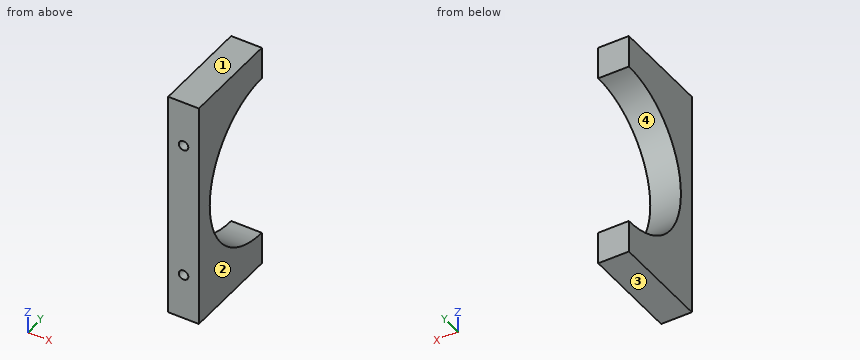
Autodesk Inventor part; units mm, degrees
ref_plane "YZ Plane" through (0, 0, 0) normal (1, 0, 0) x (0, 1, 0)
ref_plane "XZ Plane" through (0, 0, 0) normal (0, 1, 0) x (-1, 0, 0)
ref_plane "XY Plane" through (0, 0, 0) normal (0, 0, 1) x (1, 0, 0)
sketch "스케치1" plane through (0, 0, 0) normal (1, 0, 0) x (0, 1, 0)
  line L0 (0, 0) -> (27, 0)
  line L1 (27, -60) -> (0, -60)
  line L2 (0, -60) -> (0, 0)
  arc A0 (27, -8.5) -> (27, -51.5) centre (27, -30) ccw
  line L3 (27, 0) -> (27, -8.5)
  line L4 (27, -51.5) -> (27, -60)
  dimension "d0" = 27
  dimension "d3" = 60
  dimension "d4" = 27
  dimension "d5" = 21.5
  dimension "d6" = 27
  dimension "d7" = 30
extrude "돌출1" add sketch "스케치1" along normal blind 8
sketch "스케치2" plane through (0, 0, -60) normal (0, -1, 0) x (1, 0, 0)
  line L0 (0, 0) -> (0, 60)
  line L1 (0, 0) -> (8, 0)
  line L2 (8, 60) -> (8, 0)
  line L3 (0, 60) -> (8, 60)
  line L4 (0, 60) -> (0, 51.5)
  line L5 (0, 60) -> (8, 60)
  line L6 (8, 51.5) -> (8, 60)
  line L7 (0, 51.5) -> (8, 51.5)
  line L8 (0, 8.5) -> (0, 0)
  line L9 (0, 8.5) -> (8, 8.5)
  line L10 (8, 0) -> (8, 8.5)
  line L11 (0, 0) -> (8, 0)
  circle A0 centre (4, 48) radius 1.25
  circle A1 centre (4, 12) radius 1.25
  dimension "d10" = 2.5
  dimension "d11" = 2.5
  dimension "d12" = 4
  dimension "d13" = 4
  dimension "d14" = 12
  dimension "d15" = 12
extrude "돌출2" cut sketch "스케치2" against normal blind 9 contours A0 | A1
sketch "스케치3" plane through (0, 0, -60) normal (0, -1, 0) x (1, 0, 0)
  circle A0 centre (4, 48) radius 1.25
  circle A1 centre (4, 12) radius 1.25
  line L0 (0, 0) -> (0, 60)
  line L1 (0, 0) -> (8, 0)
  line L2 (8, 60) -> (8, 0)
  line L3 (0, 60) -> (8, 60)
extrude "돌출3" cut sketch "스케치3" against normal blind 1
properties part number "모터받침대" material "ABS 플라스틱"
CAD build for the part. Positions are in the model's coordinates, mm. Face numbers are marked on the shaded views. Coordinates: 2 decimals unless noted, no trailing zeros. Write each loop counter-clockwise with the first axis right and the second up, starting at its lowest first coordinate (ties: lowest second). Pieces come first, ordered by that corner, then holes. Notation, with made-up numbers: (68, 40.25) -> (87, 40.25) arc R23 ccw to (87, 65.25) -> close; hole circle Ø5 at (-27.75, 13.5). An arc over 180 degrees is marked (long way). Return JSON: item names as keys, results as strings. Group by question number.
Q1. Cut at C-C, the plane z = -12. Give the cut face in (x, y).
Q2. Flat gauge pins, fed straight in: pin 1 (2 mm diameter, centred on x = 2.5, y = 23, fed in from +Z); pin 2 (2 mm diameter, centred on x = 4, z = -48, fed in from +Y); pin 3 (0.8 mm diameter, centred on x = 4, z = -47.5, fed in from -Y). Where does each tip first touch, or does it go through?
Q3. Drill centre lines: line 1 (Z direction, x = 4, y = 3.25); line 2 (Z direction, x = 4, y = 7.25); line 3 (Z direction, x = 7.75, y = 24.5). Where is each one in solid material? Low to high.
Q4. Cut at B-B, the plane x = 1.25. Give the cut face in (y, z).
Q5. Cut at D-D, the plane y = 24.75. Give the cut face in (x, z), then the cut area to 3 significant figures.
Q6. Cut at A-A, the plane y = 20.5. Give the cut face in (x, z), then the cut area to 3 significant figures.
Q7. Pull direction Z, two halves, no side cores. Call the marked faces 1, 2, 3 and 4: released by +Z, released by -Z, zero draft, split by the parting line, or undercut.
Returned:
{
 "1": {"outline": "(0, 1) -> (2.75, 1) -> (2.75, 9) -> (5.25, 9) -> (5.25, 1) -> (8, 1) -> (8, 15.24) -> (0, 15.24) -> close"},
 "2": {"pin 1": "stops at z = 0", "pin 2": "stops at y = 16.94", "pin 3": "stops at y = 9"},
 "3": {"line 1": "z = -60 to -49.25, -46.75 to -13.25, -10.75 to 0", "line 2": "z = -60 to -49.25, -46.75 to -38.5, -21.5 to -13.25, -10.75 to 0", "line 3": "z = -60 to -51.35, -8.65 to 0"},
 "4": {"outline": "(1, -60) -> (27, -60) -> (27, -51.5) arc R21.5 cw to (27, -8.5) -> (27, 0) -> (1, 0) -> close"},
 "5": {"outline": "(0, -60) -> (8, -60) -> (8, -51.38) -> (0, -51.38) -> close; (0, -8.62) -> (8, -8.62) -> (8, 0) -> (0, 0) -> close", "area": "138 mm2"},
 "6": {"outline": "(0, -60) -> (8, -60) -> (8, -50.49) -> (0, -50.49) -> close; (0, -9.51) -> (8, -9.51) -> (8, 0) -> (0, 0) -> close", "area": "152 mm2"},
 "7": {"face 1": "released by +Z", "face 2": "zero draft", "face 3": "released by -Z", "face 4": "undercut"}
}
